Read the model definition and answer for the solid it produces. Units are mm, in the model's axes. Face numbers are marked on the shaded views. A direction names the side the tool comes from. Give positions to 0.01 mm unless a question says otherwise; leave off trailing zeros. Answer as a JSON object with one key per item and string values. Group by question number.
```python
from build123d import *

# Parameters (mm, degrees)
EXTRUDE_1_DEPTH          = 36
CUT_EXTRUDE_START        = 4
SKETCH_2_R               = 6
CUT_EXTRUDE_1_DEPTH      = 32
SKETCH_2_3_R             = 7.5
CUT_EXTRUDE_2_DEPTH      = 32
PATTERN_CIRCULAR_1_COUNT = 3
EXTRUDE_START            = -4
EXTRUDE_2_DEPTH          = 4
FILLET_1_R               = 5
SKETCH_7_W               = 2
SKETCH_7_H               = 6
SKETCH_8_R               = 1.55
CUT_EXTRUDE_4_DEPTH      = 8
CUT_EXTRUDE_START_2      = -1
SKETCH_11_W              = 5.6
SKETCH_11_H              = 2.6
CUT_EXTRUDE_5_DEPTH      = 79.193153111
SKETCH_12_R              = 5
CUT_EXTRUDE_7_DEPTH      = 1.5
SKETCH_13_R              = 6
CUT_EXTRUDE_8_DEPTH      = 3
PATTERN_CIRCULAR_3_COUNT = 3
SKETCH_14_R              = 8.7
SKETCH_14_R_2            = 7.2
CUT_EXTRUDE_9_DEPTH      = 2
PATTERN_CIRCULAR_4_COUNT = 3
PATTERN_CIRCULAR_5_COUNT = 3


with BuildPart() as part:
    # Sketch 3 → Extrude 1 (new body)
    with BuildSketch(Plane.XY):
        with BuildLine():
            Line((11.835680518, 43.594010768), (-11.835680518, 43.594010768))
            Line((-11.835680518, 43.594010768), (-23.253520778, 23.817731326))
            ThreePointArc((-23.253520778, 23.817731326), (-19.959292144, 20.523502692), (-18.753520778, 16.023502692))
            ThreePointArc((-18.753520778, 16.023502692), (-23.253520778, 8.229274058), (-32.253520778, 8.229274058))
            Line((-32.253520778, 8.229274058), (-43.671361037, -11.547005384))
            Line((-43.671361037, -11.547005384), (-31.835680518, -32.047005384))
            Line((-31.835680518, -32.047005384), (-9, -32.047005384))
            ThreePointArc((-9, -32.047005384), (0, -23.047005384), (9, -32.047005384))
            Line((9, -32.047005384), (31.835680518, -32.047005384))
            Line((31.835680518, -32.047005384), (43.671361037, -11.547005384))
            Line((43.671361037, -11.547005384), (32.253520778, 8.229274058))
            ThreePointArc((32.253520778, 8.229274058), (19.959292144, 11.523502692), (23.253520778, 23.817731326))
            Line((23.253520778, 23.817731326), (11.835680518, 43.594010768))
        make_face()
    extrude(amount=EXTRUDE_1_DEPTH)

    # Sketch 2 → Cut-Extrude 1 (cut)
    # profile 1 of 2: a face of its own
    with BuildSketch(Plane.XY.offset(CUT_EXTRUDE_START)):
        with BuildLine():
            ThreePointArc((-10.207581819, 15.879076713), (-8.566497102, 11.096786669), (-9.762812095, 6.184324194))
            Line((-9.762812095, 6.184324194), (-10.237187905, 5.362681189))
            ThreePointArc((-10.237187905, 5.362681189), (-13.893347706, 1.870410777), (-18.855474732, 0.90048681))
            ThreePointArc((-18.855474732, 0.90048681), (-10.765375864, -3.122534061), (-7.5, -11.547005384))
            ThreePointArc((-7.5, -11.547005384), (-7.790345243, -14.225499495), (-8.647892913, -16.779563523))
            ThreePointArc((-8.647892913, -16.779563523), (-5.326850604, -12.967197446), (-0.47437581, -11.547005384))
            Line((-0.47437581, -11.547005384), (0.47437581, -11.547005384))
            ThreePointArc((0.47437581, -11.547005384), (5.326850604, -12.967197446), (8.647892913, -16.779563523))
            ThreePointArc((8.647892913, -16.779563523), (9.174682453, -5.297005384), (18.855474732, 0.90048681))
            ThreePointArc((18.855474732, 0.90048681), (13.893347706, 1.870410777), (10.237187905, 5.362681189))
            Line((10.237187905, 5.362681189), (9.762812095, 6.184324194))
            ThreePointArc((9.762812095, 6.184324194), (8.566497102, 11.096786669), (10.207581819, 15.879076713))
            ThreePointArc((10.207581819, 15.879076713), (0, 10.594010768), (-10.207581819, 15.879076713))
        make_face()
        Circle(SKETCH_2_R, mode=Mode.SUBTRACT)
    # profile 2 of 2: a face of its own
    with BuildSketch(Plane.XY.offset(CUT_EXTRUDE_START)):
        Circle(SKETCH_2_R)
    extrude(amount=CUT_EXTRUDE_1_DEPTH, mode=Mode.SUBTRACT)

    # Sketch 2_3 → Cut-Extrude 2 (cut)
    # profile 1 of 6: a face of its own
    with BuildSketch(Plane.XY.offset(CUT_EXTRUDE_START)):
        with BuildLine():
            ThreePointArc((12.5, 23.094010768), (-3.785183434, 35.007129015), (-10.207581819, 15.879076713))
            ThreePointArc((-10.207581819, 15.879076713), (0, 10.594010768), (10.207581819, 15.879076713))
            ThreePointArc((10.207581819, 15.879076713), (11.913118247, 19.308827333), (12.5, 23.094010768))
        make_face()
        with Locations((0, 23.094010768)):
            Circle(SKETCH_2_3_R, mode=Mode.SUBTRACT)
    # profile 2 of 6: a face of its own
    with BuildSketch(Plane.XY.offset(CUT_EXTRUDE_START)):
        with Locations((0, 23.094010768)):
            Circle(SKETCH_2_3_R)
    # profile 3 of 6: a face of its own
    with BuildSketch(Plane.XY.offset(CUT_EXTRUDE_START)):
        with BuildLine():
            ThreePointArc((-7.5, -11.547005384), (-10.765375864, -3.122534061), (-18.855474732, 0.90048681))
            ThreePointArc((-18.855474732, 0.90048681), (-30.825317547, -17.797005384), (-8.647892913, -16.779563523))
            ThreePointArc((-8.647892913, -16.779563523), (-7.790345243, -14.225499495), (-7.5, -11.547005384))
        make_face()
        with Locations((-20, -11.547005384)):
            Circle(SKETCH_2_3_R, mode=Mode.SUBTRACT)
    # profile 4 of 6: a face of its own
    with BuildSketch(Plane.XY.offset(CUT_EXTRUDE_START)):
        with Locations((-20, -11.547005384)):
            Circle(SKETCH_2_3_R)
    # profile 5 of 6: a face of its own
    with BuildSketch(Plane.XY.offset(CUT_EXTRUDE_START)):
        with BuildLine():
            ThreePointArc((32.5, -11.547005384), (28.424471323, -2.312381248), (18.855474732, 0.90048681))
            ThreePointArc((18.855474732, 0.90048681), (9.174682453, -5.297005384), (8.647892913, -16.779563523))
            ThreePointArc((8.647892913, -16.779563523), (22.678494112, -23.756660141), (32.5, -11.547005384))
        make_face()
        with Locations((20, -11.547005384)):
            Circle(SKETCH_2_3_R, mode=Mode.SUBTRACT)
    # profile 6 of 6: a face of its own
    with BuildSketch(Plane.XY.offset(CUT_EXTRUDE_START)):
        with Locations((20, -11.547005384)):
            Circle(SKETCH_2_3_R)
    extrude(amount=CUT_EXTRUDE_2_DEPTH, mode=Mode.SUBTRACT)

    # Sketch 4 → Cut-Revolve 1 (revolve, cut)
    with BuildSketch(Plane(origin=(0, 0, 0), x_dir=(0, 0, -1), z_dir=(1, 0, 0))):
        with BuildLine():
            ThreePointArc((-5, 35.594010768), (-2.897363718, 38.9251472), (0, 41.594010768))
            Line((0, 41.594010768), (0, 23.094010768))
            Line((0, 23.094010768), (-5, 23.094010768))
            Line((-5, 23.094010768), (-5, 35.594010768))
        make_face()
    cut_revolve_1 = revolve(axis=Axis((0, 23.094010768, 0), (0, 0, 1)), mode=Mode.SUBTRACT)

    # Pattern Circular 1: Cut-Revolve 1 ×3 about axis
    pattern_circular_1_axis = Axis((0, 0, 0), (0, 0, 1))
    for i in range(1, PATTERN_CIRCULAR_1_COUNT):
        add(cut_revolve_1.rotate(pattern_circular_1_axis, i * 360 / PATTERN_CIRCULAR_1_COUNT), mode=Mode.SUBTRACT)

    # Sketch 3_3 → Extrude 2 (add)
    with BuildSketch(Plane.XY.offset(EXTRUDE_START)):
        with BuildLine():
            Line((11.835680518, 43.594010768), (-11.835680518, 43.594010768))
            Line((-11.835680518, 43.594010768), (-23.253520778, 23.817731326))
            ThreePointArc((-23.253520778, 23.817731326), (-19.959292144, 20.523502692), (-18.753520778, 16.023502692))
            ThreePointArc((-18.753520778, 16.023502692), (-23.253520778, 8.229274058), (-32.253520778, 8.229274058))
            Line((-32.253520778, 8.229274058), (-43.671361037, -11.547005384))
            Line((-43.671361037, -11.547005384), (-31.835680518, -32.047005384))
            Line((-31.835680518, -32.047005384), (-9, -32.047005384))
            ThreePointArc((-9, -32.047005384), (0, -23.047005384), (9, -32.047005384))
            Line((9, -32.047005384), (31.835680518, -32.047005384))
            Line((31.835680518, -32.047005384), (43.671361037, -11.547005384))
            Line((43.671361037, -11.547005384), (32.253520778, 8.229274058))
            ThreePointArc((32.253520778, 8.229274058), (19.959292144, 11.523502692), (23.253520778, 23.817731326))
            Line((23.253520778, 23.817731326), (11.835680518, 43.594010768))
        make_face()
    extrude(amount=EXTRUDE_2_DEPTH)

    # Fillet 1
    fillet_1_edges = [part.edges().sort_by_distance(p)[0] for p in [
        (-9, -32.047005384, 16),
        (-31.835680518, -32.047005384, 16),
        (-43.671361037, -11.547005384, 16),
        (-32.253520778, 8.229274058, 16),
        (-23.253520778, 23.817731326, 16),
        (-11.835680518, 43.594010768, 16),
        (11.835680518, 43.594010768, 16),
        (23.253520778, 23.817731326, 16),
        (32.253520778, 8.229274058, 16),
        (43.671361037, -11.547005384, 16),
        (31.835680518, -32.047005384, 16),
        (9, -32.047005384, 16),
    ]]
    fillet(fillet_1_edges, radius=FILLET_1_R)

    # Sweep 1: sweep along a path in Sketch 6
    with BuildLine(Plane.XY.offset(36)) as sweep_1_path:
        Line((-13.808144519, 13.177602903), (-18.316211134, 5.369402481))
        ThreePointArc((-18.316211134, 5.369402481), (-19.620040628, 4.002917019), (-21.405510065, 3.387000825))
        ThreePointArc((-21.405510065, 3.387000825), (-32.990381057, -19.047005384), (-7.769526275, -20.23121591))
        ThreePointArc((-7.769526275, -20.23121591), (-6.343392486, -18.992912117), (-4.508066615, -18.547005384))
        Line((-4.508066615, -18.547005384), (4.508066615, -18.547005384))
        ThreePointArc((4.508066615, -18.547005384), (6.343392486, -18.992912117), (7.769526275, -20.23121591))
        ThreePointArc((7.769526275, -20.23121591), (32.990381057, -19.047005384), (21.405510065, 3.387000825))
        ThreePointArc((21.405510065, 3.387000825), (19.620040628, 4.002917019), (18.316211134, 5.369402481))
        Line((18.316211134, 5.369402481), (13.808144519, 13.177602903))
        ThreePointArc((13.808144519, 13.177602903), (13.276648142, 14.989995098), (13.63598379, 16.844215085))
        ThreePointArc((13.63598379, 16.844215085), (0, 38.094010768), (-13.63598379, 16.844215085))
        ThreePointArc((-13.63598379, 16.844215085), (-13.276648142, 14.989995098), (-13.808144519, 13.177602903))
    # Sketch 7 → Sweep 1 (sweep, cut)
    with BuildSketch(Plane(origin=(0, 0, 0), x_dir=(0, 1, 0), z_dir=(-1, 0, 0))):
        with Locations((38.094010768, -36)):
            Rectangle(SKETCH_7_W, SKETCH_7_H)
    sweep(path=sweep_1_path.line, mode=Mode.SUBTRACT)

    # Sketch 8 → Cut-Extrude 4 (cut)
    with BuildSketch(Plane.XY.offset(36)):
        with Locations((-13.423393759, 7.75)):
            Circle(SKETCH_8_R)
        with Locations((13.423393759, 7.75)):
            Circle(SKETCH_8_R)
        with Locations((0, -15.5)):
            Circle(SKETCH_8_R)
    extrude(amount=-CUT_EXTRUDE_4_DEPTH, mode=Mode.SUBTRACT)

    # Sketch 11 → Cut-Extrude 5 (cut, through all)
    with BuildSketch(Plane(origin=(0, -12.4, 0), x_dir=(1, 0, 0), z_dir=(0, 1, 0)).offset(CUT_EXTRUDE_START_2)):
        with Locations((0, -29.330246335)):
            Rectangle(SKETCH_11_W, SKETCH_11_H)
    cut_extrude_5 = extrude(amount=-CUT_EXTRUDE_5_DEPTH, mode=Mode.SUBTRACT)

    # Sketch 12 → Cut-Extrude 7 (cut)
    with BuildSketch(Plane.XY.offset(4)):
        Circle(SKETCH_12_R)
    extrude(amount=-CUT_EXTRUDE_7_DEPTH, mode=Mode.SUBTRACT)

    # Sketch 13 → Cut-Extrude 8 (cut)
    with BuildSketch(Plane.XY):
        with Locations((-20, -11.547005384)):
            Circle(SKETCH_13_R)
    cut_extrude_8 = extrude(amount=-CUT_EXTRUDE_8_DEPTH, mode=Mode.SUBTRACT)

    # Pattern Circular 3: Cut-Extrude 8 ×3 about axis
    pattern_circular_3_axis = Axis((0, 0, 0), (0, 0, 1))
    for i in range(1, PATTERN_CIRCULAR_3_COUNT):
        add(cut_extrude_8.rotate(pattern_circular_3_axis, i * 360 / PATTERN_CIRCULAR_3_COUNT), mode=Mode.SUBTRACT)

    # Sketch 14 → Cut-Extrude 9 (cut)
    with BuildSketch(Plane.XY):
        with Locations((-20, -11.547005384)):
            Circle(SKETCH_14_R)
        with Locations((-20, -11.547005384)):
            Circle(SKETCH_14_R_2, mode=Mode.SUBTRACT)
    cut_extrude_9 = extrude(amount=-CUT_EXTRUDE_9_DEPTH, mode=Mode.SUBTRACT)

    # Pattern Circular 4: Cut-Extrude 9 ×3 about axis
    pattern_circular_4_axis = Axis((0, 0, 0), (0, 0, 1))
    for i in range(1, PATTERN_CIRCULAR_4_COUNT):
        add(cut_extrude_9.rotate(pattern_circular_4_axis, i * 360 / PATTERN_CIRCULAR_4_COUNT), mode=Mode.SUBTRACT)

    # Pattern Circular 5: Cut-Extrude 5 ×3 about axis
    pattern_circular_5_axis = Axis((0, 0, 0), (0, 0, 1))
    for i in range(1, PATTERN_CIRCULAR_5_COUNT):
        add(cut_extrude_5.rotate(pattern_circular_5_axis, i * 360 / PATTERN_CIRCULAR_5_COUNT), mode=Mode.SUBTRACT)


solid = part.part
```
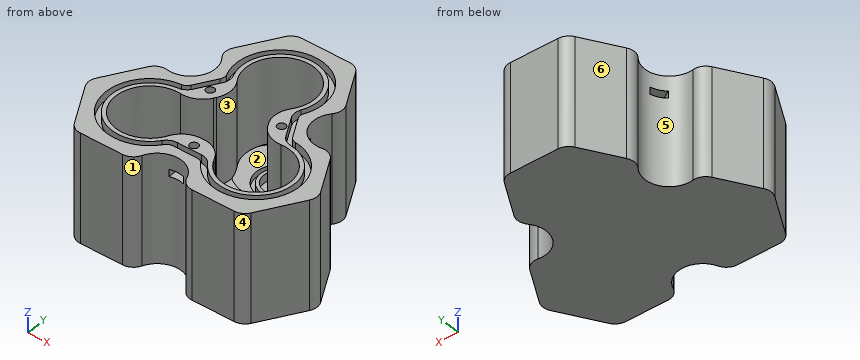
1) Flat-ended cylindrical pins translate along their axes: pin 1 Ø5 at (y, z) = (19, 26) entering from +X; pin 2 Ø8 at (y, z) = (10.5, 17) entering from -X; pin 3 Ø8.5 at (x, y) = (-23.5, -15.5) entering from +Z. Find the tip coordinate at first contact, or state that the pin passes through.
2) For a pull along Y with two mould halves and no side action, classify the marked faces 4, 5 and 6 as released by +Y, released by -Y, zero draft, split by the parting line, or undercut.
3) Find the intervals of material crossed by line 1 (Y direction, x = -20, z = 22); line 2 (Y direction, x = -20, z = -1); line 3 (X direction, y = -13, z = 27), in increasing order. Write a range as [from, to].
4) Which of the six approach directions +Z, -Z, +X, -X, +Y, -Y give full straight-line access (tool end or side, diameter ignored) to the marked faces 1, 2 and 3?
Values follow:
{
 "1": {"pin 1": "stops at x = 20.61", "pin 2": "stops at x = -32.51", "pin 3": "stops at z = 0"},
 "2": {"face 4": "released by -Y", "face 5": "undercut", "face 6": "released by +Y"},
 "3": {"line 1": "y = [-32.05, -24.05], [0.95, 11.45], [20.59, 29.45]", "line 2": "y = [-32.05, -20.25], [-18.75, -17.55], [-5.55, -4.35], [-2.85, 11.45], [20.59, 29.45]", "line 3": "x = [-42.68, -32.42], [-5.38, 5.38], [32.42, 42.68]"},
 "4": {"face 1": "+Z, -Z, -Y", "face 2": "none", "face 3": "+Z"}
}
